CAD build for the part. Positions are in the model's coordinates, mm. A direction names the side the tool comes from. Round coordinates to 2 decimals unless told otherwise and drop trailing zeros. Order: outer loops, then holes, each group sorted by start corner. A loop starts at its lowest first (then second) coordinate and runs counter-clockwise, first axis right, second up. Notation, with made-up numbers: M -15.5,70.25 L 4.5,70.25 A26 ccw 4.5,100.25 Z; hole C 78,87 d2. An arc over 180 degrees is marked long. Answer as a JSON object with one key per item and string values.
Autodesk Inventor part; units mm, degrees
ref_plane "YZ Plane" through (0, 0, 0) normal (1, 0, 0) x (0, 1, 0)
ref_plane "XZ Plane" through (0, 0, 0) normal (0, 1, 0) x (-1, 0, 0)
ref_plane "XY Plane" through (0, 0, 0) normal (0, 0, 1) x (1, 0, 0)
sketch "Sketch1" plane through (0, 0, 0) normal (1, 0, 0) x (0, 1, 0)
  line L0 (0, 0) -> (20, 0)
  line L1 (20, 0) -> (20, -7)
  line L2 (20, -7) -> (0, -7)
  line L3 (0, -7) -> (0, 0)
  dimension "d18" = 20
  dimension "d19" = 7
extrude "Extrusion1" add sketch "Sketch1" along normal blind 20
sketch "Sketch2" plane through (0, 8.5, -7) normal (0, 0, -1) x (-1, 0, 0)
  line L0 (0, 11.5) -> (0, 0)
  line L1 (0, 11.5) -> (-20, 11.5)
  line L2 (-20, 0) -> (-20, 11.5)
  line L3 (0, 0) -> (-20, 0)
  line L4 (0, 11.5) -> (-20, 11.5)
  line L5 (-10, 11.5) -> (-10, 5.5)
  circle A0 centre (-10, 5.5) radius 2.2
  line L6 (0, 11.5) -> (-20, 11.5)
  point P0 (0, -8.5)
  dimension "d6" = 6
  dimension "d7" = 4.4
extrude "Extrusion2" cut sketch "Sketch2" against normal through all contours A0
sketch "Sketch11" plane through (0, 0, -7) normal (0, -1, 0) x (1, 0, 0)
  line L0 (0, 0) -> (20, 0)
  line L1 (10, 0) -> (17.2, 0)
  line L2 (20, 7) -> (20, 0)
  arc A0 (17.2, -11) -> (25.2, -3) centre (17.2, -3) ccw
  line L3 (10, 0) -> (10, -11)
  line L4 (17.2, -11) -> (10, -11)
  line L5 (25.2, 7) -> (25.2, -3)
  circle A1 centre (17.2, -3) radius 2.2
  line L6 (0, 7) -> (20, 7)
  line L7 (25.2, 7) -> (20, 7)
  line L8 (20, 7) -> (20, 10)
  line L9 (20, 10) -> (25.2, 7)
  line L10 (17.2, -3) -> (17.2, 7)
  point P0 (13.4, 7)
  dimension "d58" = 7.2
  dimension "d66" = 4.4
  dimension "d72" = 3
  dimension "d73" = 10
  dimension "d75" = 8
extrude "Extrusion10" add sketch "Sketch11" against normal blind 7 contours L0 L2 L7 L5 A0 L4 L3 | L8 L9 L7
sketch "Sketch14" plane through (0, 7, -7) normal (0, 1, 0) x (1, 0, 0)
  circle A0 centre (17.2, 3) radius 2.2
  circle A1 centre (17.2, 3) radius 3.6
  point P0 (0, -7)
  dimension "d76" = 7.2
extrude "Extrusion11" cut sketch "Sketch14" along normal through all
mirror "Mirror4" about plane through (10, 0, -18) normal (-1, 0, 0) of "Extrusion10", "Extrusion11"
fillet "Fillet3" radius 2.8 1 edges at (10, 20, -7)
chamfer "Chamfer1" distance 3 angle 45 5 edges at (10, 7, -18) (-2.8569, 7, -15.6569) (-5.2, 7, -5) (22.8569, 7, -15.6569) (25.2, 7, -5)
sketch "Sketch15" plane through (0, 20, 0) normal (0, 0, 1) x (1, 0, 0)
  circle A0 centre (10, -6) radius 2.2
  line L0 (10, -6) -> (10, -10.4)
  line L1 (2.8, -20) -> (17.2, -20)
  line L2 (7.5, -10.4) -> (12.5, -10.4)
  line L3 (12.5, -10.4) -> (12.5, -20)
  line L4 (12.5, -20) -> (7.5, -20)
  line L5 (7.5, -20) -> (7.5, -10.4)
  point P0 (0, -20)
  dimension "d83" = 4.4
  dimension "d84" = 5
extrude "Extrusion12" add sketch "Sketch15" along normal blind 1.6 contours L2 L3 L1 L5
fillet "Fillet4" radius 0.4 2 edges at (12.5, 4.8, 0) (7.5, 4.8, 0)
properties part number "Ljoint"
Item 1: Saw through at A-A on z = 0.75. List the corners of the cut face in (x, y).
Worked answers:
{"outline": "M -3.9,0 L 0,0 L 0,7 L -2.2,7 L -3.9,5.3 Z; M 7.5,0 L 12.5,0 L 12.5,9.6 L 7.5,9.6 Z; M 20,0 L 23.9,0 L 23.9,5.3 L 22.2,7 L 20,7 Z"}
Item 2: Drop flat-ended pins along their axis: pin 1 Ø0.8 at (x, z) = (11, 0.5) entering from +Y; pin 2 Ø1.5 at (x, z) = (5.5, -14.5) entering from +Y; pin 3 Ø1 at (x, y) = (10, 9) entering from +Z; pin 4 Ø4 at (x, z) = (17.2, -10) entering from +Y. Give the stop position or say it passes through.
Worked answers:
{"pin 1": "stops at y = 9.6", "pin 2": "stops at y = 7", "pin 3": "stops at z = 1.6", "pin 4": "passes through"}
Item 3: 3-axis set-ups, long thin cutter, end or side, ignore diameter. For faces 1 (the flat face through (0, 13, -3)), 2 (the flat face through (12.5, 5, 1)), 3 (the cylindrical face through (17.2, 12.9, -6.4)): which of +Z, -Z, +X, -X, +Y, -Y reach the whole face in a straight line?
Worked answers:
{"face 1": "+Z, -Z, -X, +Y", "face 2": "+Z, +Y, -Y", "face 3": "-Z, +Y"}
Item 4: Saw through at B-B on z = -1.75. List the corners of the cut face in (x, y).
Worked answers:
{"outline": "M -5.2,0 L 25.2,0 L 25.2,4 L 22.2,7 L 20,7 L 20,20 L 0,20 L 0,7 L -2.2,7 L -5.2,4 Z; hole C 10,14 d4.4"}
Item 5: Two-plate mould, pull along X, no slides. Class faces 4 (the conical face through (21.53, 5.81, -14.42)), 5 (the flat face through (10, 9.6, 1)), 6 (the cylindrical face through (2.8, 12.9, -6.4)): released by +X, released by -X, zero draft, split by the parting line, or undercut.
Worked answers:
{"face 4": "released by +X", "face 5": "zero draft", "face 6": "undercut"}
Item 6: Wall check: line 1 along X through (y, z) = (2.25, -10); line 2 along Z through (x, y) = (17.2, 4); line 3 along X through (y, z) = (5.75, -10). Give the ranges that are in metal, low to high. Write a range as [from, to].
Worked answers:
{"line 1": "x = [-5.2, 0.6], [5, 15], [19.4, 25.2]", "line 2": "z = [-18, -12.2], [-7.8, 0]", "line 3": "x = [-3.45, 0.6], [5, 15], [19.4, 23.45]"}
Item 7: Saw through at C-C on y = 14. List the corners of the cut face in (x, z).
Worked answers:
{"outline": "M 0,-7 L 0.81,-7 A3.6 cw 4.79,-7 L 7.8,-7 L 7.8,0 L 0,0 Z; M 12.2,-7 L 15.21,-7 A3.6 cw 19.19,-7 L 20,-7 L 20,0 L 12.2,0 Z"}
